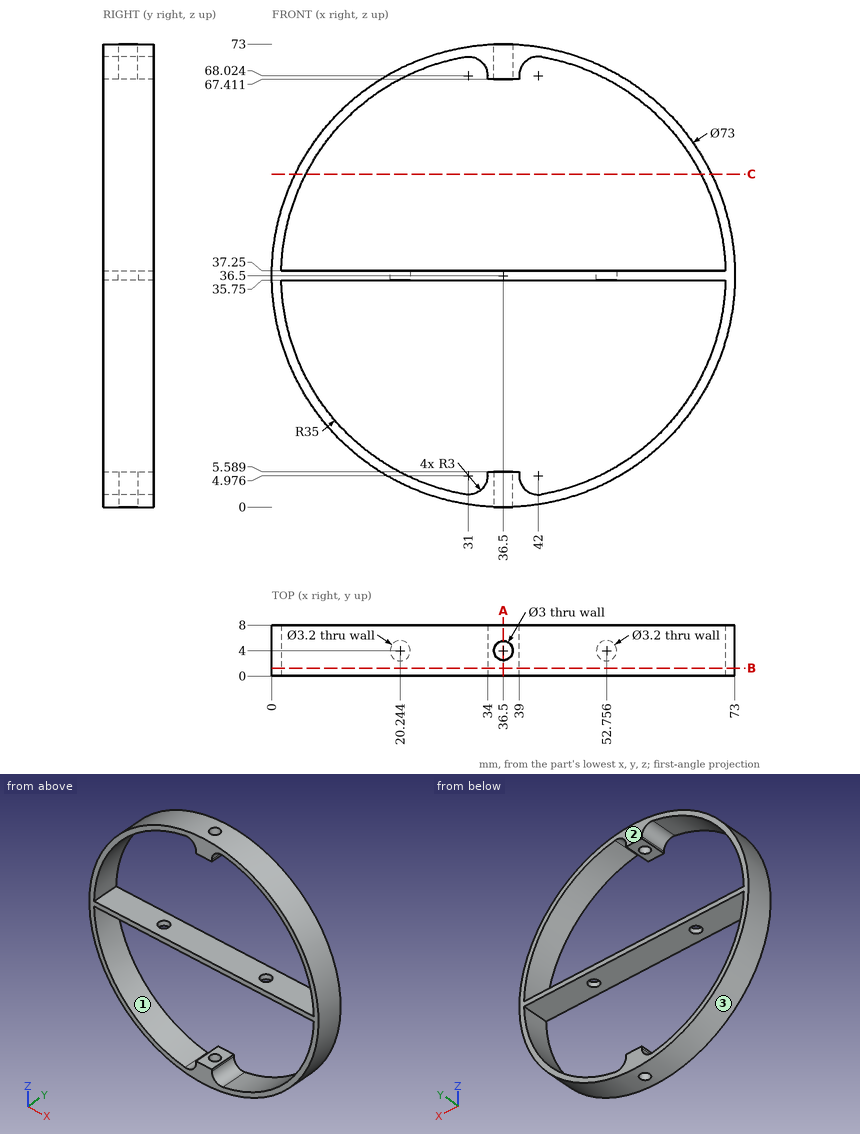
Input: dimensioned drawing with shaded views. Units: mm. Origin: part minimum x, y, z. Round coordinates to 2 decimals unless told otherwise and drop trailing zeros. Order: outer loops, then holes, each group sorted by start corner. A loop starts at its lowest first (then second) coordinate and runs counter-clockwise, first axis right, second up.
Q1. Section C-C, the plane z = 52.5. Output: boundary loops of the cut face in (x, y).
Result sheet:
outline: (3.69, 0) - (5.37, 0) - (5.37, 8) - (3.69, 8) - close; (67.63, 0) - (69.31, 0) - (69.31, 8) - (67.63, 8) - close
Q2. Pin query (flat end, axial travel): pin 1 (0.7 mm diameter, centred on y = 4.5, z = 67.5, fed in from +X); pin 2 (0.7 mm diameter, centred on y = 5.5, z = 67.5, fed in from -X); pin 3 (3 mm diameter, centred on x = 52.756, y = 4, fed in from +Z) (1 decimal). Return the tip coordinate at first contact, or that it passes through.
Result sheet:
pin 1: stops at x = 56.32
pin 2: stops at x = 16.68
pin 3: stops at z = 69.9
Q3. Material intervals for probe 1 along Z at (x, y) = (37.5, 2.25); probe 2 along Z at (x, y) = (31, 3.5); probe 3 along Y at (x, z) = (36.5, 70.85), sorted ascending.
Result sheet:
probe 1: z = 0.01 to 5.59, 35.75 to 37.25, 67.41 to 72.99
probe 2: z = 0.42 to 1.98, 35.75 to 37.25, 71.02 to 72.58
probe 3: y = 0 to 2.5, 5.5 to 8
Q4. Section A-A, the plane x = 36.5. Output: boundary loops of the cut face in (y, z).
Result sheet:
outline: (0, 0) - (2.5, 0) - (2.5, 5.59) - (0, 5.59) - close; (0, 35.75) - (8, 35.75) - (8, 37.25) - (0, 37.25) - close; (0, 67.41) - (2.5, 67.41) - (2.5, 73) - (0, 73) - close; (5.5, 0) - (8, 0) - (8, 5.59) - (5.5, 5.59) - close; (5.5, 67.41) - (8, 67.41) - (8, 73) - (5.5, 73) - close
Q5. Mould query, pull axis Z, two halves, no side actions, for the marked faces 1, 2 and 3. Classes: released by +Z, released by -Z, zero draft, split by the parting line, or undercut.
Result sheet:
face 1: undercut
face 2: zero draft
face 3: split by the parting line
Q6. Section B-B, the plane y = 1.25. Give the number of separate pieces and of enclosed holes in the cut face.
Result sheet:
separate pieces: 1
enclosed holes: 2
